Can you work these out from the model? Positions are in its coordinate system, mm. Face numbers are marked on the shaded views. A direction names the side the tool comes from. Give positions to 0.01 mm unless a question says otherwise; leave off trailing zeros. Loops run counter-clockwise (first coordinate to the right, second up) from the corner with the lowest first, then second, coordinate; pieces in that order, holes last.
from build123d import *

# Parameters (mm, degrees)
CROQUIS1_R                         = 1.6
BASE_TAPA_DEPTH                    = 3
CROQUIS2_R                         = 1.5
SOPORTES_TAPA_DEPTH                = 8
CROQUIS3_R                         = 3.5
CAJA_HORN_SERVO_EXTERIOR_1_DEPTH   = 4
CROQUIS4_R                         = 0.75
CAJA_HORN_SERVO_EXTERIOR_2_DEPTH   = 2
CROQUIS5_R                         = 0.75
TALADROS_HORN_SERVO_EXTERIOR_DEPTH = 4
CROQUIS6_R                         = 1.5
TALADROS_TAPA_DEPTH                = 11
CROQUIS7_R                         = 1.6
RECTIFICAR_TALADRO_DEPTH           = 3
CHAFL_N_TALADROS_TAPA_SIZE         = 1


with BuildPart() as part:
    # Croquis1 → Base Tapa (new body)
    with BuildSketch(Plane.XY):
        with BuildLine():
            Line((11.548443784, 19.3588474), (-11.785521088, 19.3588474))
            ThreePointArc((-11.785521088, 19.3588474), (-41.605177571, 9.733322379), (-31.246229762, -19.839551086))
            Line((-31.246229762, -19.839551086), (-31.246229762, -38.896936565))
            Line((-31.246229762, -38.896936565), (31.339101257, -38.896936565))
            Line((31.339101257, -38.896936565), (31.339101257, -19.919367151))
            ThreePointArc((31.339101257, -19.919367151), (41.646982557, 9.899296763), (11.548443784, 19.3588474))
        make_face()
        with Locations((-22, 0)):
            Circle(CROQUIS1_R, mode=Mode.SUBTRACT)
        with Locations((22, 0)):
            Circle(CROQUIS1_R, mode=Mode.SUBTRACT)
    extrude(amount=BASE_TAPA_DEPTH)

    # Croquis2 → Soportes tapa (add)
    with BuildSketch(Plane.XY.offset(3)):
        with BuildLine():
            ThreePointArc((-31.246229762, -34.896936565), (-30.074656886, -37.725363689), (-27.246229762, -38.896936565))
            Line((-27.246229762, -38.896936565), (27.339101257, -38.896936565))
            ThreePointArc((27.339101257, -38.896936565), (30.167528382, -37.725363689), (31.339101257, -34.896936565))
            Line((31.339101257, -34.896936565), (31.339101257, -26.154350822))
            Line((31.339101257, -26.154350822), (27.339101257, -26.154350822))
            Line((27.339101257, -26.154350822), (27.339101257, -30.896936565))
            ThreePointArc((27.339101257, -30.896936565), (24.510674133, -32.06850944), (23.339101257, -34.896936565))
            Line((23.339101257, -34.896936565), (-23.246229762, -34.896936565))
            ThreePointArc((-23.246229762, -34.896936565), (-24.417802637, -32.06850944), (-27.246229762, -30.896936565))
            Line((-27.246229762, -30.896936565), (-27.246229762, -26.154350822))
            Line((-27.246229762, -26.154350822), (-31.246229762, -26.154350822))
            Line((-31.246229762, -26.154350822), (-31.246229762, -34.896936565))
        make_face()
        with Locations((-27.246229762, -34.896936565)):
            Circle(CROQUIS2_R, mode=Mode.SUBTRACT)
        with Locations((27.339101257, -34.896936565)):
            Circle(CROQUIS2_R, mode=Mode.SUBTRACT)
        with BuildLine():
            Line((7.423794942, 19.3588474), (-7.423794942, 19.3588474))
            ThreePointArc((-7.423794942, 19.3588474), (-3.142422422, 15.219148939), (0, 10.160252288))
            ThreePointArc((0, 10.160252288), (3.142422422, 15.219148939), (7.423794942, 19.3588474))
        make_face()
        with Locations((0, 16.857587951)):
            Circle(CROQUIS2_R, mode=Mode.SUBTRACT)
    extrude(amount=SOPORTES_TAPA_DEPTH)

    # Croquis3 → Caja Horn servo exterior 1 (cut)
    with BuildSketch(Plane(origin=(0, -34.896936565, 0), x_dir=(1, 0, 0), z_dir=(0, 1, 0))):
        with Locations((0, -7)):
            Circle(CROQUIS3_R)
    extrude(amount=-CAJA_HORN_SERVO_EXTERIOR_1_DEPTH, mode=Mode.SUBTRACT)

    # Croquis4 → Caja Horn servo exterior 2 (cut)
    with BuildSketch(Plane.XZ.offset(38.896936565)):
        with BuildLine():
            Line((-16, 9.5), (-5.123475383, 11))
            ThreePointArc((-5.123475383, 11), (0, 13.5), (5.123475383, 11))
            Line((5.123475383, 11), (16, 9.5))
            ThreePointArc((16, 9.5), (18.5, 7), (16, 4.5))
            Line((16, 4.5), (5.123475383, 3))
            ThreePointArc((5.123475383, 3), (0, 0.5), (-5.123475383, 3))
            Line((-5.123475383, 3), (-16, 4.5))
            ThreePointArc((-16, 4.5), (-18.5, 7), (-16, 9.5))
        make_face()
        with Locations((-16, 7)):
            Circle(CROQUIS4_R, mode=Mode.SUBTRACT)
        with Locations((-13, 7.017965487)):
            Circle(CROQUIS4_R, mode=Mode.SUBTRACT)
        with Locations((-10.006253635, 6.991538598)):
            Circle(CROQUIS4_R, mode=Mode.SUBTRACT)
        with Locations((-7.006253635, 7.009504085)):
            Circle(CROQUIS4_R, mode=Mode.SUBTRACT)
        with Locations((7.006253635, 7.009504085)):
            Circle(CROQUIS4_R, mode=Mode.SUBTRACT)
        with Locations((10.006253635, 6.991538598)):
            Circle(CROQUIS4_R, mode=Mode.SUBTRACT)
        with Locations((13, 7.017965487)):
            Circle(CROQUIS4_R, mode=Mode.SUBTRACT)
        with Locations((16, 7)):
            Circle(CROQUIS4_R, mode=Mode.SUBTRACT)
    extrude(amount=-CAJA_HORN_SERVO_EXTERIOR_2_DEPTH, mode=Mode.SUBTRACT)

    # Croquis5 → Taladros Horn servo exterior (cut)
    with BuildSketch(Plane.XZ.offset(38.896936565)):
        with Locations((-16, 7)):
            Circle(CROQUIS5_R)
        with Locations((-13, 7.017965487)):
            Circle(CROQUIS5_R)
        with Locations((-10.006253635, 6.991538598)):
            Circle(CROQUIS5_R)
        with Locations((-7.006253635, 7.009504085)):
            Circle(CROQUIS5_R)
        with Locations((7.006253635, 7.009504085)):
            Circle(CROQUIS5_R)
        with Locations((10.006253635, 6.991538598)):
            Circle(CROQUIS5_R)
        with Locations((13, 7.017965487)):
            Circle(CROQUIS5_R)
        with Locations((16, 7)):
            Circle(CROQUIS5_R)
    extrude(amount=-TALADROS_HORN_SERVO_EXTERIOR_DEPTH, mode=Mode.SUBTRACT)

    # Croquis6 → Taladros Tapa (cut)
    with BuildSketch(Plane.XY.offset(11)):
        with Locations((0, 16.857587951)):
            Circle(CROQUIS6_R)
        with Locations((27.339101257, -34.896936565)):
            Circle(CROQUIS6_R)
        with Locations((-27.246229762, -34.896936565)):
            Circle(CROQUIS6_R)
    extrude(amount=-TALADROS_TAPA_DEPTH, mode=Mode.SUBTRACT)

    # Croquis7 → Rectificar taladro (add)
    with BuildSketch(Plane.XY.offset(3)):
        with Locations((-22, 0)):
            Circle(CROQUIS7_R)
    extrude(amount=-RECTIFICAR_TALADRO_DEPTH)

    # Chaflán taladros tapa
    chafl_n_taladros_tapa_edges = [part.edges().sort_by_distance(p)[0] for p in [
        (-1.5, 16.857587951, 0),
        (25.839101257, -34.896936565, 0),
        (-28.746229762, -34.896936565, 0),
    ]]
    chamfer(chafl_n_taladros_tapa_edges, length=CHAFL_N_TALADROS_TAPA_SIZE)


solid = part.part
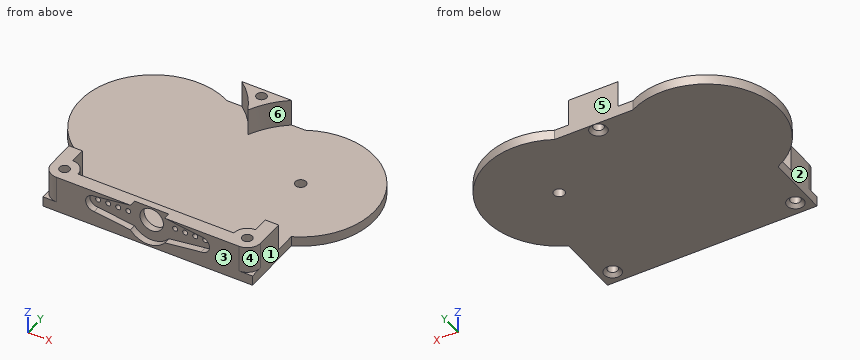
(1) Please list where these lines run through material, in increasing order: probe 1 along Z at (x, y) = (16, -36); probe 2 along Z at (x, y) = (0, -36); probe 3 along Z at (x, y) = (10, -13.5).
Returned:
probe 1: z = 0 to 6.25, 7.75 to 11
probe 2: z = 0 to 3.5, 10.5 to 11
probe 3: z = 0 to 3
(2) Which directions (+Z, -Z, +X, -X, +Y, -Y) give clear straight access to the entire face, cutting with the end or side of a thin tool? Please do the marked faces 1, 2 and 3.
Returned:
face 1: +Z, -Z, +X, -Y
face 2: +Z, -Z, -X, -Y
face 3: +Z, -Z, +X, -X, -Y
(3) Thinking about a two-plate mould opening in Y: for the marked faces 4, 5 and 6, which applies, pulls with the +Y half, pulls with the -Y half, needs draft (parallel to the pull), parting line crosses it, or undercut?
Returned:
face 4: pulls with the -Y half
face 5: pulls with the +Y half
face 6: undercut
(4) Suppose I cut it at D-D on x = -22. List the corners of the cut face in (y, z) for me.
Returned:
outline: (-38.9, 0) - (21.89, 0) - (21.89, 3) - (-34.9, 3) - (-34.9, 11) - (-38.9, 11) - close
(5) Suppose I cut it at B-B on z = 2. List the corners of the cut face in (x, y) for me.
Returned:
outline: (-31.25, -38.9) - (-4.15, -38.9) - (-4.15, -36.9) - (4.15, -36.9) - (4.15, -38.9) - (31.34, -38.9) - (31.34, -19.92) arc R22 ccw (long way) to (11.55, 19.36) - (-11.79, 19.36) arc R21.89 ccw (long way) to (-31.25, -19.84) - close; hole circle Ø3 at (-27.25, -34.9); hole circle Ø3 at (0, 16.86); hole circle Ø3.2 at (22, 0); hole circle Ø3 at (27.34, -34.9)
(6) Will these pins go through, and if not, where does the flat tip stop? P1, Ø3, axis at x = -29.5, z = 7.5, coming from the +Y side; P2, Ø1, axis at x = -8, y = 12.5, coming from the +Z side; P3, Ø1, axis at x = 28.5, z = 1.5, coming from the +Y side; P4, Ø4, axis at x = 22, y = 0, coming from the -Z side.
Returned:
P1: stops at y = -26.15
P2: stops at z = 3
P3: stops at y = 21.17
P4: stops at z = 0
(7) Suppose I cut it at A-A on x = 22. List the corners of the cut face in (y, z) for me, plus the area to 3 significant figures.
Returned:
outline: (-38.9, 0) - (-1.6, 0) - (-1.6, 3) - (-34.9, 3) - (-34.9, 11) - (-38.9, 11) - close; (1.6, 0) - (22, 0) - (22, 3) - (1.6, 3) - close
area: 205 mm2
(8) Suppose I cut it at C-C on y = 12. List the corners of the cut face in (x, z) for me, plus the area to 3 significant figures.
Returned:
outline: (-40.31, 0) - (40.44, 0) - (40.44, 3) - (0.95, 3) - (0.95, 11) - (-0.95, 11) - (-0.95, 3) - (-40.31, 3) - close
area: 257 mm2
